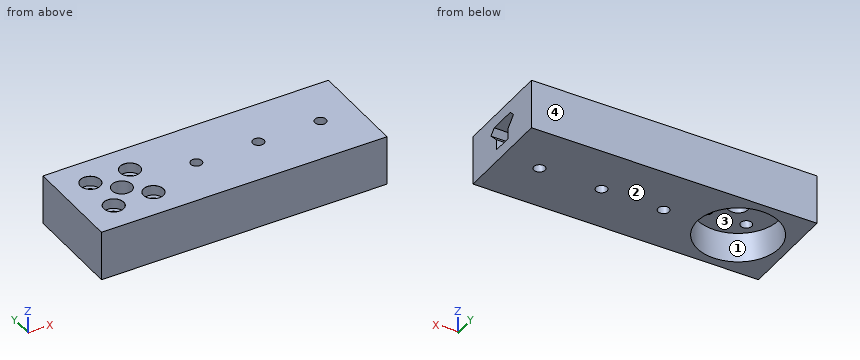
```python
from build123d import *

# Parameters (mm, degrees)
SKETCH1_W                     = 115
SKETCH1_H                     = 40
SKETCH1_R                     = 4
BOSS_EXTRUDE1_DEPTH           = 10
CBORE_FOR_M4_SHCS1_AT_2_COUNT = 2
CBORE_FOR_M4_SHCS1_AT_2_PITCH = 16
CBORE_FOR_M4_SHCS1_AT_3_COUNT = 2
CBORE_FOR_M4_SHCS1_AT_3_PITCH = 16
CBORE_FOR_M4_SHCS1_AT_4_COUNT = 2
CBORE_FOR_M4_SHCS1_AT_4_PITCH = 22.627416998
SKETCH5_R                     = 16.5
SKETCH5_R_2                   = 4
CUT_EXTRUDE1_DEPTH            = 12
CUT_EXTRUDE2_DEPTH            = 75
M4_CLEARANCE_HOLE1_D          = 4.5


with BuildPart() as part:
    # Sketch1 → Boss-Extrude1 (new body, symmetric)
    with BuildSketch(Plane.XY):
        with Locations((17.5, 0)):
            Rectangle(SKETCH1_W, SKETCH1_H)
        with Locations((-20, 0)):
            Circle(SKETCH1_R, mode=Mode.SUBTRACT)
    extrude(amount=BOSS_EXTRUDE1_DEPTH, both=True)

    # Sketch3 → CBORE for M4 SHCS1 (revolve, cut)
    with BuildSketch(Plane(origin=(-28, 8, 10), x_dir=(0, -1, 0), z_dir=(1, 0, 0))):
        Polygon((0, 0), (0, 20), (2.25, 20), (2.25, 4), (4, 4), (4, 0.025), (4.025, 0), align=None)
    cbore_for_m4_shcs1 = revolve(axis=Axis((-28, 8, 16.35), (0, 0, -1)), mode=Mode.SUBTRACT)

    # CBORE for M4 SHCS1 at 2: CBORE for M4 SHCS1 ×2
    with Locations(*[(i * CBORE_FOR_M4_SHCS1_AT_2_PITCH, 0, 0) for i in range(1, CBORE_FOR_M4_SHCS1_AT_2_COUNT)]):
        add(cbore_for_m4_shcs1, mode=Mode.SUBTRACT)

    # CBORE for M4 SHCS1 at 3: CBORE for M4 SHCS1 ×2
    with Locations(*[(0, -i * CBORE_FOR_M4_SHCS1_AT_3_PITCH, 0) for i in range(1, CBORE_FOR_M4_SHCS1_AT_3_COUNT)]):
        add(cbore_for_m4_shcs1, mode=Mode.SUBTRACT)

    # CBORE for M4 SHCS1 at 4: CBORE for M4 SHCS1 ×2
    with Locations(*[Vector(0.707106781, -0.707106781, 0) * (i * CBORE_FOR_M4_SHCS1_AT_4_PITCH) for i in range(1, CBORE_FOR_M4_SHCS1_AT_4_COUNT)]):
        add(cbore_for_m4_shcs1, mode=Mode.SUBTRACT)

    # Sketch5 → Cut-Extrude1 (cut)
    with BuildSketch(Plane(origin=(0, 0, -10), x_dir=(-1, 0, 0), z_dir=(0, 0, -1))):
        with Locations((20, 0)):
            Circle(SKETCH5_R)
        with Locations((20, 0)):
            Circle(SKETCH5_R_2, mode=Mode.SUBTRACT)
    extrude(amount=-CUT_EXTRUDE1_DEPTH, mode=Mode.SUBTRACT)

    # Sketch6 → Cut-Extrude2 (cut)
    with BuildSketch(Plane(origin=(75, 0, 0), x_dir=(0, 0, -1), z_dir=(1, 0, 0))):
        Polygon((-5.1, 5.5), (-2.9, 7.7), (0.8, 4), (5.1, 4), (5.1, 0), (-5.1, 0), align=None)
    cut_extrude2 = extrude(amount=-CUT_EXTRUDE2_DEPTH, mode=Mode.SUBTRACT)

    # Mirror1: Cut-Extrude2 across plane
    add(cut_extrude2.mirror(Plane(origin=(-12.780062598, 0, 5.1), x_dir=(0, 0, 1), z_dir=(0, -1, 0))), mode=Mode.SUBTRACT)

    # M4 Clearance Hole1 (through all)
    with Locations(Plane(origin=(0, 0, -10), x_dir=(-1, 0, 0), z_dir=(0, 0, -1))):
        with Locations((-10, 0), (-35, 0), (-60, 0)):
            Hole(M4_CLEARANCE_HOLE1_D / 2)


solid = part.part
```
The listing builds one solid part. Answer for the finished solid, in the listing's coordinates (mm). Face numbers are marked on the shaded views. Give positions to 0.01 mm unless a question says otherwise; leave off trailing zeros. Loops run counter-clockwise (first coordinate to the right, second up) from the corner with the lowest first, then second, coordinate; pieces in that order, holes last. Notation, with made-up numbers: M 80,72 L 91,72 A24 cw 91,108 Z; hole C 54.5,4.5 d6. An arc over 180 degrees is marked long. One line per item, written item: value.
Q1. A cutting plane is placed at C-C on x = 24.5. Determine the outline of the cut face in (y, z), then the cut area to 3 significant figures.
Working result:
outline: M -20,-10 L 20,-10 L 20,10 L -20,10 Z; hole M -7.7,2.9 L -4,-0.8 L -4,-5.1 L 4,-5.1 L 4,-0.8 L 7.7,2.9 L 5.5,5.1 L -5.5,5.1 Z
area: 693 mm^2
Q2. A cutting plane is placed at A-A on x = 10. Determine the outline of the cut face in (y, z), then the cut area to 3 significant figures.
Working result:
outline: M -20,-10 L -2.25,-10 L -2.25,-5.1 L -4,-5.1 L -4,-0.8 L -7.7,2.9 L -5.5,5.1 L -2.25,5.1 L -2.25,10 L -20,10 Z; M 2.25,-10 L 20,-10 L 20,10 L 2.25,10 L 2.25,5.1 L 5.5,5.1 L 7.7,2.9 L 4,-0.8 L 4,-5.1 L 2.25,-5.1 Z
area: 649 mm^2
Q3. Determine the mould class of the marked faces 1, 2, 3 and 4 for opening direction Y: +Y half, -Y half, draft (parallel to the pull), parting line (faces both ways), or undercut.
Working result:
face 1: undercut
face 2: draft
face 3: undercut
face 4: +Y half
Q4. A cutting plane is placed at D-D on z = 4. Determine the outline of the cut face in (x, y), then the cut area to 3 significant figures.
Working result:
outline: M -40,-20 L 75,-20 L 75,-6.6 L 0,-6.6 L 0,6.6 L 75,6.6 L 75,20 L -40,20 Z; hole C -28,-8 d4.5; hole C -28,8 d4.5; hole C -20,0 d8; hole C -12,-8 d4.5; hole C -12,8 d4.5
area: 3,500 mm^2
Q5. Flat-ended cylindrical pins translate along their axes: P1, Ø4, axis at x = -11.5, y = 7, coming from the +Z side; P2, Ø20, axis at x = -20, y = 0, coming from the -Z side. Find the tip coordinate at first contact, or state that the pin passes through.
Working result:
P1: stops at z = 6
P2: stops at z = 2
Q6. Find the intervals of material crossed by line 1 (X direction, y = -8, z = 2.9); line 2 (X direction, y = 8, z = 8.7); line 3 (Y direction, x = -28, z = 4.7), in increasing order. Write a range as from..to.
Working result:
line 1: x = -40..-30.25, -25.75..-14.25, -9.75..75
line 2: x = -40..-32, -24..-16, -8..75
line 3: y = -20..-10.25, -5.75..5.75, 10.25..20
Q7. A cutting plane is placed at B-B on z = -8.25. Determine the outline of the cut face in (x, y).
Working result:
outline: M -40,-20 L 75,-20 L 75,20 L -40,20 Z; hole C -20,0 d33; hole C 10,0 d4.5; hole C 35,0 d4.5; hole C 60,0 d4.5
